```python
from build123d import *

# Parameters (mm, degrees)
BOSS_EXTRUDE1_DEPTH = 6
SKETCH2_W           = 21
SKETCH2_H           = 7
SKETCH2_W_2         = 13
SKETCH2_H_2         = 20
CUT_EXTRUDE1_DEPTH  = 91.752410436
SKETCH3_R           = 1
CUT_EXTRUDE2_DEPTH  = 91.752410436


with BuildPart() as part:
    # Sketch1 → Boss-Extrude1 (new body)
    with BuildSketch(Plane(origin=(0, 0, 0), x_dir=(1, 0, 0), z_dir=(0, 1, 0))):
        Polygon((33, 32), (66, 32), (66, 28), (60, 28), (60, 24), (66, 24), (66, 20), (60, 20), (60, 16), (66, 16), (66, 12), (60, 12), (60, 8), (66, 8), (66, 4), (60, 4), (60, 0), (0, 0), (0, 20), (0, 62), (33, 62), align=None)
    extrude(amount=BOSS_EXTRUDE1_DEPTH)

    # Sketch2 → Cut-Extrude1 (cut, through all)
    with BuildSketch(Plane(origin=(0, 6, 0), x_dir=(1, 0, 0), z_dir=(0, 1, 0))):
        with Locations((16.5, 9.5)):
            Rectangle(SKETCH2_W, SKETCH2_H)
        with Locations((16.5, 42)):
            Rectangle(SKETCH2_W_2, SKETCH2_H_2)
    extrude(amount=-CUT_EXTRUDE1_DEPTH, mode=Mode.SUBTRACT)

    # Sketch3 → Cut-Extrude2 (cut, through all)
    with BuildSketch(Plane(origin=(0, 6, 0), x_dir=(1, 0, 0), z_dir=(0, 1, 0))):
        with Locations(Location((64, 30, 0), (0, 0, 270))):
            Circle(SKETCH3_R)
        with Locations(Location((64, 22, 0), (0, 0, 270))):
            Circle(SKETCH3_R)
        with Locations(Location((64, 14, 0), (0, 0, 270))):
            Circle(SKETCH3_R)
        with Locations(Location((64, 6, 0), (0, 0, 270))):
            Circle(SKETCH3_R)
        with Locations((60, 26)):
            Circle(SKETCH3_R)
        with Locations((60, 18)):
            Circle(SKETCH3_R)
        with Locations((60, 10)):
            Circle(SKETCH3_R)
        with Locations((60, 2)):
            Circle(SKETCH3_R)
    extrude(amount=-CUT_EXTRUDE2_DEPTH, mode=Mode.SUBTRACT)


solid = part.part
```
The model under review builds one solid part; all positions refer to its coordinate system, in mm. A direction names the side the tool comes from. Coordinates: 2 decimals unless noted, no trailing zeros. Write each loop counter-clockwise with the first axis right and the second up, starting at its lowest first coordinate (ties: lowest second). Pieces come first, ordered by that corner, then holes.
1) We need section C-C on z = -35. State the section outline as (x, y) points.
2) The part is to be moulded in two halves that separate along X. For faces 1 (the face through (66, 3, -30)), 2 (the face through (64.84, 3.04, -13.46)), 3 (the face through (49, 3, -32)), say which applies: pulls with the +X half, pulls with the -X half, needs draft (parallel to the pull), parting line crosses it, or undercut.
3) To check wall thickness, follow probe 1 along Z at (x, y) = (19, 5.25); probe 2 along X at (y, z) = (2.15, -14); probe 3 along X at (y, z) = (5, -45.5). State the ranges of each line that lie inside material, in increasing order.
4) We need section D-D on y = 4.5. Count the separate pieces of the cut face and the enclosed holes in it, then the cut area to 3 significant figures.
5) We need section B-B on z = -10. State the section outline as (x, y) points.
6) Clearance check with flat-ended pins moving along their axes: pin 1 Ø0.8 at (y, z) = (1.5, -19.5) entering from +X; pin 2 Ø1.8 at (x, y) = (63, 3) entering from -Z; pin 3 Ø1.8 at (x, z) = (64, -22) entering from +Y; pin 4 Ø1.8 at (y, z) = (3.5, -54.5) entering from +X. State where each tip first meets the part, or that it passes through.
7) We need section A-A on x = 20.5. State the section outline as (y, z) points.
8) Machinability: for faces 4 (the face through (33, 3, -47)), 5 (the face through (16, 3, -32)), 6 (the face through (63, 3, -20)), 7 (the face through (26, 6, -25)), which of the approach directions +Z, -Z, +X, -X, +Y, -Y give a long, thin tool a straight path to every point of the face, cutting with its end or side? Answer none if there is none.
Answer list:
1. outline: (0, 0) - (10, 0) - (10, 6) - (0, 6) - close; (23, 0) - (33, 0) - (33, 6) - (23, 6) - close
2. face 1: pulls with the +X half
2. face 2: undercut
2. face 3: needs draft
3. probe 1: z = -62 to -52, -32 to -13, -6 to 0
3. probe 2: x = 0 to 63, 65 to 66
3. probe 3: x = 0 to 10, 23 to 33
4. separate pieces: 1
4. enclosed holes: 6
4. area: 2,580 mm2
5. outline: (0, 0) - (6, 0) - (6, 6) - (0, 6) - close; (27, 0) - (59, 0) - (59, 6) - (27, 6) - close
6. pin 1: stops at x = 60
6. pin 2: stops at z = -32
6. pin 3: passes through
6. pin 4: stops at x = 33
7. outline: (0, -62) - (6, -62) - (6, -52) - (0, -52) - close; (0, -32) - (6, -32) - (6, -13) - (0, -13) - close; (0, -6) - (6, -6) - (6, 0) - (0, 0) - close
8. face 4: -Z, +X, +Y, -Y
8. face 5: +Y, -Y
8. face 6: +X, +Y, -Y
8. face 7: +Z, -Z, +X, -X, +Y
